For this review, use the dimensioned drawing (mm, ordinates from the lowest corner) and the shaded views. Give positions to 0.01 mm unless a question says otherwise; leave off trailing zeros. Order: outer loops, then holes, each group sorted by start corner. A loop starts at its lowest first (then second) coordinate and runs counter-clockwise, first axis right, second up.
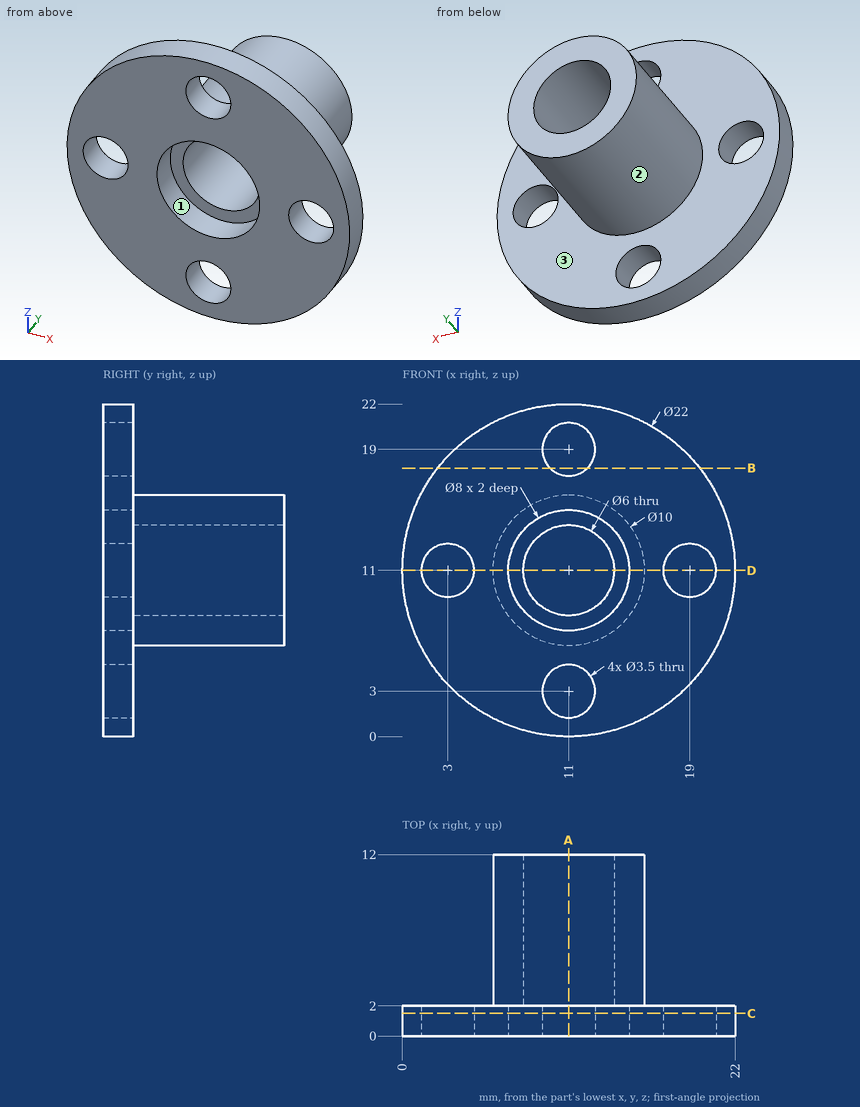
1. For line 1 along X through (y, z) = (0.95, 11); line 2 along X through (y, z) = (6.75, 11); line 3 along Y through (x, z) = (13.75, 9), list the stretches that pass through material, from the lowest coordinate up.
Recorded:
line 1: x = 0 to 1.25, 4.75 to 7, 15 to 17.25, 20.75 to 22
line 2: x = 6 to 8, 14 to 16
line 3: y = 2 to 12
2. For pin 1 (3 mm diameter, centred on x = 19, z = 11, fed in from +Y); pin 2 (3 mm diameter, centred on y = 10, z = 16, fed in from +X); pin 3 (3 mm diameter, centred on x = 5.5, y = 8, fed in from -Z); pin 4 (2 mm diameter, centred on x = 10.5, y = 10.5, fed in from +Z), all flat-tipped, find the tip position at first contact; note any pin that passes through.
Recorded:
pin 1: passes through
pin 2: stops at x = 14.57
pin 3: stops at z = 8
pin 4: stops at z = 16
3. Draft analysis for pull direction X (two halves, no side actions). For the marked faces 1, 2 and 3, state which applies: pulls with the +X half, pulls with the -X half, needs draft (parallel to the pull), parting line crosses it, or undercut.
Recorded:
face 1: undercut
face 2: parting line crosses it
face 3: needs draft
4. Take a section at C-C (y = 1.5). State the section outline as (x, z) points, then the cut area to 3 significant figures.
Recorded:
outline: circle Ø22 at (11, 11); hole circle Ø3.5 at (3, 11); hole circle Ø8 at (11, 11); hole circle Ø3.5 at (11, 3); hole circle Ø3.5 at (11, 19); hole circle Ø3.5 at (19, 11)
area: 291 mm2
5. Take a section at A-A (x = 11). State the section outline as (y, z) points, then the cut area to 3 significant figures.
Recorded:
outline: (0, 0) - (2, 0) - (2, 1.25) - (0, 1.25) - close; (0, 4.75) - (2, 4.75) - (2, 6) - (12, 6) - (12, 8) - (2, 8) - (2, 7) - (0, 7) - close; (0, 15) - (2, 15) - (2, 14) - (12, 14) - (12, 16) - (2, 16) - (2, 17.25) - (0, 17.25) - close; (0, 20.75) - (2, 20.75) - (2, 22) - (0, 22) - close
area: 54.0 mm2
6. Take a section at B-B (z = 17.75). State the section outline as (x, y) points.
Recorded:
outline: (2.31, 0) - (9.78, 0) - (9.78, 2) - (2.31, 2) - close; (12.22, 0) - (19.69, 0) - (19.69, 2) - (12.22, 2) - close
7. Take a section at D-D (z = 11). State the section outline as (x, y) points, then the cut area to 3 significant figures.
Recorded:
outline: (0, 0) - (1.25, 0) - (1.25, 2) - (0, 2) - close; (4.75, 0) - (7, 0) - (7, 2) - (8, 2) - (8, 12) - (6, 12) - (6, 2) - (4.75, 2) - close; (14, 2) - (15, 2) - (15, 0) - (17.25, 0) - (17.25, 2) - (16, 2) - (16, 12) - (14, 12) - close; (20.75, 0) - (22, 0) - (22, 2) - (20.75, 2) - close
area: 54.0 mm2
